Here's how the part is built. I have some questions about the finished solid (model axes, mm). Round coordinates to 2 decimals unless told otherwise and drop trailing zeros. Order: outer loops, then holes, each group sorted by start corner. A loop starts at its lowest first (then second) coordinate and runs counter-clockwise, first axis right, second up. Notation, with made-up numbers: M -1.75,-4.5 L 39.25,-4.5 A32 ccw 39.25,27.5 Z; hole C 75,82.25 d3. An arc over 180 degrees is marked long. Use one line per item in the form item = value. Start each with the question number.
Autodesk Inventor part; units mm, degrees
ref_plane "YZ Plane" through (0, 0, 0) normal (1, 0, 0) x (0, 1, 0)
ref_plane "XZ Plane" through (0, 0, 0) normal (0, 1, 0) x (-1, 0, 0)
ref_plane "XY Plane" through (0, 0, 0) normal (0, 0, 1) x (1, 0, 0)
sketch "Sketch1" plane through (0, 0, 0) normal (0, 1, 0) x (-1, 0, 0)
  line L0 (-38.5, 0) -> (38.5, 0)
  line L1 (27.5, 0) -> (-27.5, 0)
  line L2 (-27.5, 0) -> (-27.5, -17.5)
  line L3 (-27.5, -17.5) -> (27.5, -17.5)
  line L4 (27.5, -17.5) -> (27.5, 0)
  line L5 (0, -21) -> (0, 3.5)
  dimension "d8" = 17.5
  dimension "d22" = 55
extrude "Extrusion1" add sketch "Sketch1" along normal blind 5
sketch "Sketch2" plane through (0, 0, 0) normal (0, -1, 0) x (1, 0, 0)
  line L0 (-27.5, 0) -> (27.5, 0)
  line L1 (27.5, 0) -> (27.5, -17.5)
  line L2 (-27.5, -17.5) -> (-27.5, 0)
  point P0 (17.5, -9)
  point P1 (-17.5, -9)
  dimension "d9" = 9
  dimension "d23" = 10
  dimension "d24" = 10
hole "Hole1" at (17.5, 0, -9) at (-17.5, 0, -9) direction (0, 1, 0) diameter 6 end through all countersink diameter 10.4 countersink angle 90
chamfer "Chamfer1" distance 3 angle 45 2 edges at (-27.5, 2.5, 0) (27.5, 2.5, 0)
properties part number "FixedJaw"
1) Will this pin go through, and if not, where does the flat tip stop? pin 1 Ø1 at (x, z) = (19.5, -6) entering from -Y.
2) If we section it at C-C on z = -9: Write out the boundary of the cut face in (x, y), then the cut area to 3 significant figures.
3) If we section it at A-A on x = -17.5: Write out the boundary of the cut face in (y, z), then the cut area to 3 significant figures.
4) If we section it at D-D on y = 3.75: Write out the boundary of the cut face in (x, z).
5) If we mould it in two halves opening along X, with no side actions, what happens to faces 1 (the flat face through (0, 5, -9)), 2 (the conical face through (14.716, 2.062, -10.448)), 3 (the cylindrical face through (-14.838, 3.62, -10.384)), 4 (the flat face through (-26, 2.5, -1.5))? For each: +X half, -X half, draft (parallel to the pull), parting line (faces both ways), or undercut.
6) If we section it at B-B on y = 0.75: Write out the boundary of the cut face in (x, z).
7) If I drill on line 1 (X direction, y = 3.2, z = -9); line 2 (Z direction, x = 17.5, y = 3.3); line 3 (X direction, y = 1.95, z = -7.25), over which ranges is the centre line in solid material (lowest first)?
Completed:
q1.pin_1 = 1.09
q2.outline = M -27.5,0 L -22.7,0 L -20.5,2.2 L -20.5,5 L -27.5,5 Z; M -14.5,2.2 L -12.3,0 L 12.3,0 L 14.5,2.2 L 14.5,5 L -14.5,5 Z; M 20.5,2.2 L 22.7,0 L 27.5,0 L 27.5,5 L 20.5,5 Z
q2.area = 205 mm²
q3.outline = M 0,-17.5 L 5,-17.5 L 5,-12 L 2.2,-12 L 0,-14.2 Z; M 0,-3.8 L 2.2,-6 L 5,-6 L 5,0 L 0,0 Z
q3.area = 52.7 mm²
q4.outline = M -27.5,-17.5 L 27.5,-17.5 L 27.5,-3 L 24.5,0 L -24.5,0 L -27.5,-3 Z; hole C -17.5,-9 d6; hole C 17.5,-9 d6
q5.face_1 = draft
q5.face_2 = undercut
q5.face_3 = undercut
q5.face_4 = -X half
q6.outline = M -27.5,-17.5 L 27.5,-17.5 L 27.5,-3 L 24.5,0 L -24.5,0 L -27.5,-3 Z; hole C -17.5,-9 d8.9; hole C 17.5,-9 d8.9
q7.line_1 = -27.5 to -20.5, -14.5 to 14.5, 20.5 to 27.5
q7.line_2 = -17.5 to -12, -6 to 0
q7.line_3 = -27.5 to -20.24, -14.76 to 14.76, 20.24 to 27.5
